```python
from build123d import *

# Parameters (mm, degrees)
F1_DEPTH  = 12.7
F2_R      = 21.351508313
F5_DEPTH  = 25.4
F3_R      = 8.6303522865
F6_DEPTH  = 15.748
F7_R      = 16.3268483507
F8_DEPTH  = 25.4
F9_R      = 4.6742871789
F10_DEPTH = 25.4
F12_R     = 8.0691836116
F13_DEPTH = 6.096
F14_R     = 8.4816227384
F15_DEPTH = 6.096
F16_R     = 7.7449040589
F16_R_2   = 7.9980791945
F17_DEPTH = 9.906
F20_DEPTH = 76.2
F22_DEPTH = 54.61


with BuildPart() as f1:
    # F0 (on Top) → F1 (new body)
    with BuildSketch(Plane.XY):
        with BuildLine():
            Line((43.0717023765, 44.353062627), (-172.8282976235, 44.353062627))
            Line((-172.8282976235, 44.353062627), (-172.8282976235, -31.846937373))
            Line((-172.8282976235, -31.846937373), (43.0717023765, -31.846937373))
            ThreePointArc((43.0717023765, -31.846937373), (55.7717023765, 6.253062627), (43.0717023765, 44.353062627))
        make_face()
    extrude(amount=F1_DEPTH)

    # F2 (on face) → F5 (join)
    with BuildSketch(Plane.XY.offset(12.7)):
        with Locations((-83.9282976235, 13.9431571588)):
            Circle(F2_R)
    extrude(amount=F5_DEPTH)

    # F3 (on face) → F6 (join)
    with BuildSketch(Plane.XY.offset(12.7)):
        with Locations((17.6193086471, 10.6806947875)):
            Circle(F3_R)
    extrude(amount=F6_DEPTH)

    # F7 (on face) → F8 (cut)
    with BuildSketch(Plane.XY.offset(38.1)):
        with Locations((-83.9282976235, 13.9431571588)):
            Circle(F7_R)
    extrude(amount=-F8_DEPTH, mode=Mode.SUBTRACT)

    # F9 (on face) → F10 (cut)
    with BuildSketch(Plane.XY.offset(28.448)):
        with Locations((17.6193086471, 10.6806947875)):
            Circle(F9_R)
    extrude(amount=-F10_DEPTH, mode=Mode.SUBTRACT)

    # F12 (on face) → F13 (cut)
    with BuildSketch(Plane.XY.offset(12.7)):
        with Locations((-159.6309095621, -19.4137375802)):
            Circle(F12_R)
    extrude(amount=-F13_DEPTH, mode=Mode.SUBTRACT)

    # F14 (on face) → F15 (cut)
    with BuildSketch(Plane.XY.offset(12.7)):
        with Locations((-162.579163909, 28.7375189364)):
            Circle(F14_R)
    extrude(amount=-F15_DEPTH, mode=Mode.SUBTRACT)

    # F16 (on face) → F17 (join)
    with BuildSketch(Plane.XY.offset(12.7)):
        with Locations((-135.2781951427, 29.6167228371)):
            Circle(F16_R)
        with Locations((-135.2781951427, -19.9670530856)):
            Circle(F16_R_2)
    extrude(amount=-F17_DEPTH)

    # F19 (on face) → F20 (cut)
    with BuildSketch(Plane(origin=(-0.7380402899, 10.8379946946, 0), x_dir=(-0.9976893986, -0.0679401489, 0), z_dir=(-0.0679401489, 0.9976893986, 0))):
        Polygon((-10.0049076565, 30.4591804743), (62.7737756253, 41.8267212808), (62.7737756253, 54.864), (-10.0049076565, 54.864), align=None)
    extrude(amount=F20_DEPTH, mode=Mode.SUBTRACT)

    # F21 (on face) → F22 (cut)
    with BuildSketch(Plane(origin=(1.6560066854, 12.5212517744, 0), x_dir=(0.9913673033, -0.1311139582, 0), z_dir=(-0.1311139582, -0.9913673033, 0))):
        Polygon((7.6538164039, 54.864), (-65.4252028626, 54.864), (7.6538164039, 28.5761542618), align=None)
    extrude(amount=F22_DEPTH, mode=Mode.SUBTRACT)


solid = f1.part
```
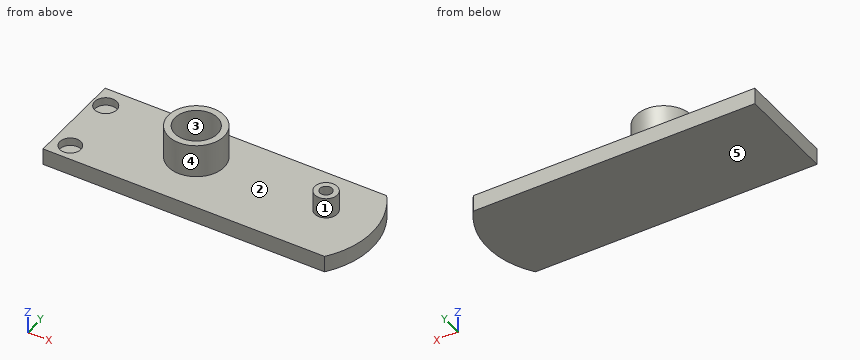
Design review of the part built by this model. Coordinates are the model's own, in mm. Face numbers are marked on the shaded views. A direction names the side the tool comes from. Coordinates: 2 decimals unless noted, no trailing zeros. Order: outer loops, then holes, each group sorted by start corner. A loop starts at its lowest first (then second) coordinate and runs counter-clockwise, first axis right, second up. Notation, with made-up numbers: M 17,0 L 42,0 A25 cw 42,19 Z; hole C 16.25,86 d1. An arc over 180 degrees is marked long. Answer as a JSON object with one key per item and string values. Group by question number.
1) Tool access review of the marked faces 4 and 5: name each direction out of +Z, -Z, +X, -X, +Y, -Y from which nothing blocks a thin tool from reaching the whole face with its end or side.
2) Add section C-C, the plane z = 24. Write out the cut boundary in (x, y), then the cut area to 3 significant figures.
3) Add section D-D, the plane y = 25. Write out the cut boundary in (x, z).
4) Wall thickness on L1, parallel to X at y = 10, z = 18; L2, parallel to Z at x = -120, y = 21.5; L3, parallel to X at y = -23, z = 10: over which ranges is each line inside the solid? List them lowest first.
5) Mouldability with a two-part tool opening along Y and no side actions: class the marked faces 1, 2 and 3 as pulls with the +Y half, pulls with the -Y half, needs draft (parallel to the pull), parting line crosses it, or undercut.
6) Add section A-A, the plane y = -24.5. Write out the cut boundary in (x, z), then the cut area to 3 significant figures.
7) Add section B-B, the plane x = -159. Write out the cut boundary in (y, z), then the cut area to 3 significant figures.
8) For pin 1 (5 mm diameter, centred on x = -160.5, y = 33, fed in from +Z); pin 2 (7.5 mm diameter, centred on x = 17.62, y = 10.68, fed in from +Z); pin 3 (19 mm diameter, centred on x = 20, y = 6.5, fed in from +Z); pin 4 (8 mm diameter, centred on y = -18, z = 20, fed in from +X), all flat-tipped, find the tip position at first contact; note any pin that passes through.
Computed values:
{
 "1": {"face 4": "+Z", "face 5": "-Z, +X, -X, +Y, -Y"},
 "2": {"outline": "C -83.93,13.94 d42.7; C 17.62,10.68 d17.26; hole C -83.93,13.94 d32.65; hole C 17.62,10.68 d9.35", "area": "760 mm^2"},
 "3": {"outline": "M -172.83,0 L 52.94,0 L 52.94,12.7 L -65.66,12.7 L -65.66,38.1 L -71.92,38.1 L -71.92,12.7 L -95.94,12.7 L -95.94,38.1 L -102.19,38.1 L -102.19,12.7 L -154.97,12.7 L -154.97,6.6 L -170.19,6.6 L -170.19,12.7 L -172.83,12.7 Z"},
 "4": {"L1": "x = -104.91 to -99.77, -68.08 to -62.94, 9.02 to 12.99, 22.24 to 26.22", "L2": "z = 0 to 12.7", "L3": "x = -172.83 to -166.86, -152.4 to 48.63"},
 "5": {"face 1": "parting line crosses it", "face 2": "needs draft", "face 3": "undercut"},
 "6": {"outline": "M -172.83,0 L 47.83,0 L 47.83,12.7 L -153.37,12.7 L -153.37,6.6 L -165.9,6.6 L -165.9,12.7 L -172.83,12.7 Z", "area": "2,730 mm^2"},
 "7": {"outline": "M -31.85,0 L 44.35,0 L 44.35,12.7 L 36.43,12.7 L 36.43,6.6 L 21.05,6.6 L 21.05,12.7 L -11.37,12.7 L -11.37,6.6 L -27.46,6.6 L -27.46,12.7 L -31.85,12.7 Z", "area": "776 mm^2"},
 "8": {"pin 1": "stops at z = 6.6", "pin 2": "stops at z = 3.05", "pin 3": "stops at z = 28.45", "pin 4": "passes through"}
}
